Geometry: see drawing. Coordinates: mm, zero at the bounding-box minimum. Coordinates: 2 decimals unless noted, no trailing zeros. Order: outer loops, then holes, each group sorted by start corner. A loop starts at its lowest first (then second) coordinate and runs counter-clockwise, first axis right, second up. Notation, with made-up numbers: M 78,34.25 L 110,34.25 A17 ccw 110,52.25 Z; hole C 65,53 d3. An arc over 180 degrees is marked long. One line per item, written item: value.
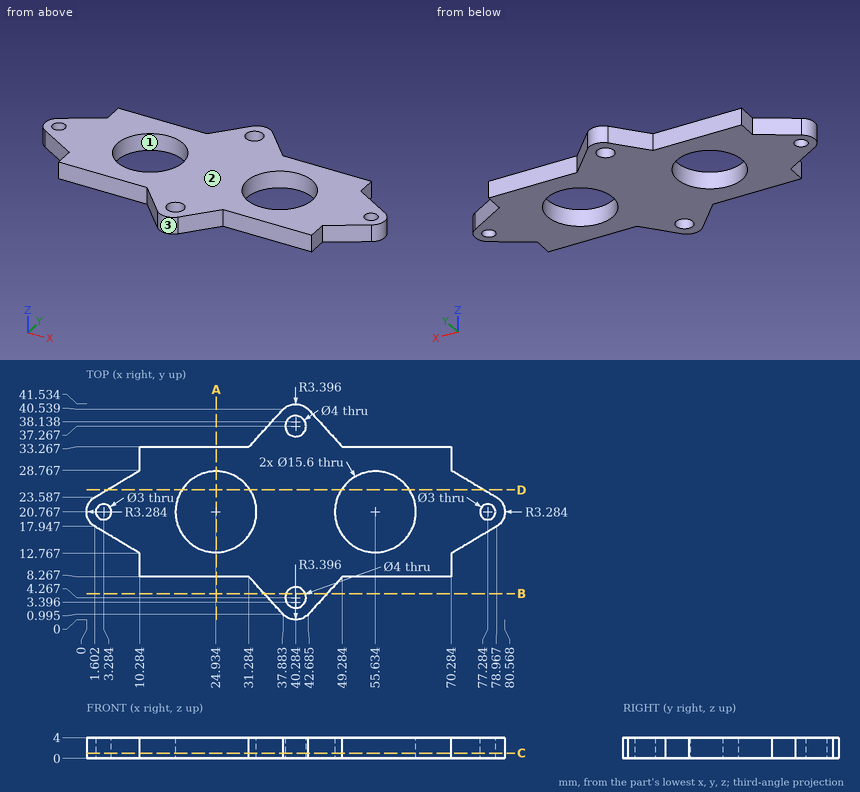
(1) Cut plane B-B on y = 5. Output: boundary loops of the cut face in (x, z) (1 decimal), plus the area to 3 significant figures.
Data:
outline: M 34.2,0 L 38.4,0 L 38.4,4 L 34.2,4 Z; M 42.1,0 L 46.3,0 L 46.3,4 L 42.1,4 Z
area: 33.4 mm2
(2) Draft query along Y for the marked faces 1, 2 and 3. Return one class per face: released by +Y, released by -Y, zero draft, split by the parting line, or undercut.
Data:
face 1: undercut
face 2: zero draft
face 3: released by -Y
(3) Cut plane C-C on z = 1. Output: boundary loops of the cut face in (x, y) (1 decimal).
Data:
outline: M 1.6,17.9 L 10.3,12.8 L 10.3,8.3 L 31.3,8.3 L 37.9,1 A3.4 ccw 42.7,1 L 49.3,8.3 L 70.3,8.3 L 70.3,12.8 L 79,17.9 A3.3 ccw 79,23.6 L 70.3,28.8 L 70.3,33.3 L 49.3,33.3 L 42.7,40.5 A3.4 ccw 37.9,40.5 L 31.3,33.3 L 10.3,33.3 L 10.3,28.8 L 1.6,23.6 A3.3 ccw Z; hole C 3.3,20.8 d3; hole C 24.9,20.8 d15.6; hole C 40.3,4.3 d4; hole C 40.3,37.3 d4; hole C 55.6,20.8 d15.6; hole C 77.3,20.8 d3
(4) Ray query, line 1 (Y direction, x = 38.5, z = 2.5) (1 decimal); line 2 (X direction, y = 27, z = 3.85) (1 decimal); line 3 (X direction, y = 19, z = 1.15) (1 decimal). Return the intervals inside material, ascending. Write a range as from..to.
Data:
line 1: y = 0.5..3.4, 5.2..36.4, 38.2..41
line 2: x = 7.3..20.2, 29.6..50.9, 60.3..73.2
line 3: x = 0.5..17.3, 32.5..48, 63.2..80.1
(5) First-contact query: pin 1 (2 mm diameter, centred on x = 55.5, z = 1, fed in from +Y); pin 2 (14 mm diameter, centred on x = 55.63, y = 20.77, fed in from -Z); pin 3 (1.5 mm diameter, centred on y = 36.5, z = 2.5, fed in from -X); pin 4 (2 mm diameter, centred on x = 22, z = 2.5, fed in from -Y). Flat tips, straight axial feed; report the tip coordinate or a pass-through.
Data:
pin 1: stops at y = 33.27
pin 2: passes through
pin 3: stops at x = 33.54
pin 4: stops at y = 8.27
(6) Cut plane D-D on y = 25. Output: boundary loops of the cut face in (x, z) (1 decimal), plus the area to 3 significant figures.
Data:
outline: M 4,0 L 18.4,0 L 18.4,4 L 4,4 Z; M 31.5,0 L 49.1,0 L 49.1,4 L 31.5,4 Z; M 62.2,0 L 76.6,0 L 76.6,4 L 62.2,4 Z
area: 186 mm2
(7) Cut plane A-A on x = 25. Output: boundary loops of the cut face in (y, z).
Data:
outline: M 8.27,0 L 12.97,0 L 12.97,4 L 8.27,4 Z; M 28.57,0 L 33.27,0 L 33.27,4 L 28.57,4 Z
